```python
from build123d import *

# Parameters (mm, degrees)
SKETCH1_W           = 20
SKETCH1_H           = 20
BOSS_EXTRUDE1_DEPTH = 20
CUT_EXTRUDE1_DEPTH  = 20
CUT_EXTRUDE2_DEPTH  = 20
CUT_EXTRUDE3_DEPTH  = 20


with BuildPart() as part:
    # Sketch1 → Boss-Extrude1 (new body)
    with BuildSketch(Plane.XY):
        with Locations((10, 10)):
            Rectangle(SKETCH1_W, SKETCH1_H)
    extrude(amount=BOSS_EXTRUDE1_DEPTH)

    # Sketch2 → Cut-Extrude1 (cut)
    with BuildSketch(Plane(origin=(0, 20, 0), x_dir=(1, 0, 0), z_dir=(0, 1, 0))):
        Polygon((20, 0), (10, 0), (20, -10), align=None)
    extrude(amount=-CUT_EXTRUDE1_DEPTH, mode=Mode.SUBTRACT)

    # Sketch3 → Cut-Extrude2 (cut)
    with BuildSketch(Plane(origin=(0, 20, 0), x_dir=(1, 0, 0), z_dir=(0, 1, 0))):
        Polygon((20, -20), (20, -10), (10, -20), align=None)
    extrude(amount=-CUT_EXTRUDE2_DEPTH, mode=Mode.SUBTRACT)

    # Sketch4 → Cut-Extrude3 (cut)
    with BuildSketch(Plane(origin=(0, 20, 0), x_dir=(1, 0, 0), z_dir=(0, 1, 0))):
        Polygon((0, 0), (10, 0), (0, -10), align=None)
    extrude(amount=-CUT_EXTRUDE3_DEPTH, mode=Mode.SUBTRACT)


solid = part.part
```
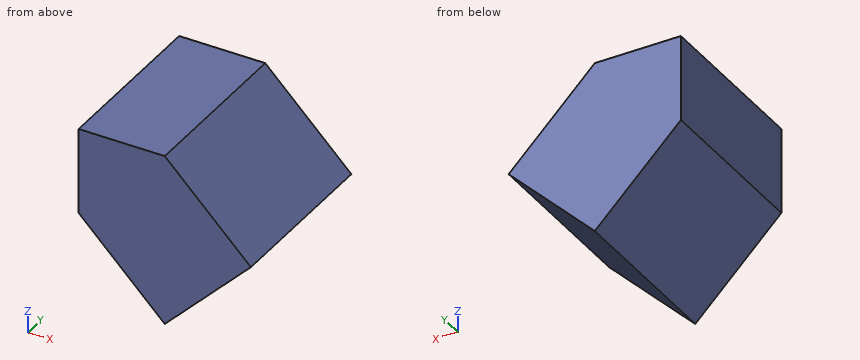
Could you check a few things on this model? Use its own coordinates, in mm. Coordinates: 2 decimals unless noted, no trailing zeros. Order: outer loops, then holes, each group sorted by start corner. A loop starts at its lowest first (then second) coordinate and runs counter-clockwise, first axis right, second up. Notation, with made-up numbers: M 38,-28 L 53,-28 A25 cw 53,-12 Z; hole C 49,32.25 d9. An arc over 180 degrees is marked long. Use a Markdown table: item, result. Add a question column.
Q1. I want a section at C-C on y = 3.5. List the corners of the cut face in (x, z) for me.
Q2. I want a section at B-B on x = 3.5. List the corners of the cut face in (y, z) for me, then the cut area to 3 significant figures.
Q3. I'm going to push flat-ended pins straight in: pin 1 (6 mm diameter, centred on x = 6.5, y = 7, fed in from -Z); pin 2 (1 mm diameter, centred on x = 14.5, y = 11.5, fed in from +Z); pin 3 (2 mm diameter, centred on y = 5.5, z = 5.5, fed in from -X). Where does each tip first touch, or does it pass through?
Q4. I want a section at A-A on z = 8. List the corners of the cut face in (x, y) for me, then the cut area to 3 significant figures.
Q5. If I drill on L1, parallel to X at y = 16.25, z = 5; L2, parallel to Z at x = 7.75, y = 16.75; L3, parallel to X at y = 13, z = 5.25, over which ranges is the centre line in solid material (lowest first)?
Checked values:
| question | item | result |
|---|---|---|
| 1 | outline | M 0,10 L 10,0 L 20,10 L 10,20 L 0,20 Z |
| 2 | outline | M 0,6.5 L 20,6.5 L 20,20 L 0,20 Z |
| 2 | area | 270 mm² |
| 3 | pin 1 | z = 0.5 |
| 3 | pin 2 | z = 16 |
| 3 | pin 3 | x = 3.5 |
| 4 | outline | M 2,0 L 18,0 L 18,20 L 2,20 Z |
| 4 | area | 320 mm² |
| 5 | L1 | 5 to 15 |
| 5 | L2 | 2.25 to 20 |
| 5 | L3 | 4.75 to 15.25 |
